Could you check a few things on this model? Use its own coordinates, in mm. A direction names the side the tool comes from. Give positions to 0.01 mm unless a question says otherwise; leave off trailing zeros. Write each loop counter-clockwise with the first axis right and the second up, starting at its lowest first coordinate (ties: lowest second). Pieces come first, ordered by that corner, then holes. Notation, with made-up numbers: (52.25, -30) - (91.25, -30) arc R19 ccw to (91.25, -4) - close; hole circle Ø6 at (-1.75, -32). An arc over 180 degrees is marked (long way). Write item = value, one per line.
from build123d import *

# Parameters (mm, degrees)
SKETCH_1_R          = 23
SKETCH_1_R_2        = 1.5
SKETCH_1_R_3        = 11.1
EXTRUDE_1_DEPTH     = 1.5
CUT_EXTRUDE_1_DEPTH = 33.56148031


with BuildPart() as part:
    # 草图1 → 凸台-拉伸1 (new body)
    with BuildSketch(Plane.XY):
        Circle(SKETCH_1_R)
        with Locations((0, 20)):
            Circle(SKETCH_1_R_2, mode=Mode.SUBTRACT)
        Circle(SKETCH_1_R_3, mode=Mode.SUBTRACT)
        with Locations((17.320508076, -10)):
            Circle(SKETCH_1_R_2, mode=Mode.SUBTRACT)
        with Locations((-17.320508076, -10)):
            Circle(SKETCH_1_R_2, mode=Mode.SUBTRACT)
    extrude(amount=EXTRUDE_1_DEPTH)

    # 草图2 → 切除-拉伸1 (cut, through all)
    with BuildSketch(Plane.XY.offset(1.5)):
        with BuildLine():
            ThreePointArc((-8.029746973, 17.219847954), (-16.454482672, 9.5), (-18.927699264, -1.655959112))
            ThreePointArc((-18.927699264, -1.655959112), (-16.815165904, -3.428585075), (-15.042539941, -1.316051715))
            ThreePointArc((-15.042539941, -1.316051715), (-13.076983597, 7.55), (-6.381535752, 13.685247584))
            ThreePointArc((-6.381535752, 13.685247584), (-5.438341178, 16.276653379), (-8.029746973, 17.219847954))
        make_face()
        with BuildLine():
            ThreePointArc((18.927699264, -1.655959112), (16.454482672, 9.5), (8.029746973, 17.219847954))
            ThreePointArc((8.029746973, 17.219847954), (5.438341178, 16.276653379), (6.381535752, 13.685247584))
            ThreePointArc((6.381535752, 13.685247584), (13.076983597, 7.55), (15.042539941, -1.316051715))
            ThreePointArc((15.042539941, -1.316051715), (16.815165904, -3.428585075), (18.927699264, -1.655959112))
        make_face()
        with BuildLine():
            ThreePointArc((-10.897952291, -15.563888841), (0, -19), (10.897952291, -15.563888841))
            ThreePointArc((10.897952291, -15.563888841), (11.376824726, -12.848068304), (8.661004189, -12.369195869))
            ThreePointArc((8.661004189, -12.369195869), (0, -15.1), (-8.661004189, -12.369195869))
            ThreePointArc((-8.661004189, -12.369195869), (-11.376824726, -12.848068304), (-10.897952291, -15.563888841))
        make_face()
    extrude(amount=-CUT_EXTRUDE_1_DEPTH, mode=Mode.SUBTRACT)


solid = part.part
1. For pin 1 (5 mm diameter, centred on x = 7, y = -1.5, fed in from +Z), with a flat end and sliding along its axis, tell me the tip position at first contact or that it passes through.
Filled sheet:
pin_1 = through
2. If we section it at A-A, the plane x = 0: Please give me the cut outline in (y, z), and give its area (4 significant figures).
Filled sheet:
outline = (-23, 0) - (-19, 0) - (-19, 1.5) - (-23, 1.5) - close; (-15.1, 0) - (-11.1, 0) - (-11.1, 1.5) - (-15.1, 1.5) - close; (11.1, 0) - (18.5, 0) - (18.5, 1.5) - (11.1, 1.5) - close; (21.5, 0) - (23, 0) - (23, 1.5) - (21.5, 1.5) - close
area = 25.35 mm2
3. If we section it at D-D, the plane z = 0.6: Please give me the cut outline in (x, y).
Filled sheet:
outline = circle Ø46 at (0, 0); hole (-18.93, -1.66) arc R1.95 ccw to (-15.04, -1.32) arc R15.1 cw to (-6.38, 13.69) arc R1.95 ccw to (-8.03, 17.22) arc R19 ccw to start; hole circle Ø3 at (-17.32, -10); hole circle Ø22.2 at (0, 0); hole (-10.9, -15.56) arc R19 ccw to (10.9, -15.56) arc R1.95 ccw to (8.66, -12.37) arc R15.1 cw to (-8.66, -12.37) arc R1.95 ccw to start; hole circle Ø3 at (0, 20); hole (6.38, 13.69) arc R15.1 cw to (15.04, -1.32) arc R1.95 ccw to (18.93, -1.66) arc R19 ccw to (8.03, 17.22) arc R1.95 ccw to start; hole circle Ø3 at (17.32, -10)
4. I need wall thicknesses on line 1 (Y direction, x = 0, z = 1.1); line 2 (Y direction, x = 9, z = 1.4); line 3 (Y direction, x = -2, z = 0.8). Which ranges of each line are inside material? Lowest first, please.
Filled sheet:
line_1 = -23 to -19, -15.1 to -11.1, 11.1 to 18.5, 21.5 to 23
line_2 = -21.17 to -16.73, -12.18 to -6.5, 6.5 to 12.12, 16.73 to 21.17
line_3 = -22.91 to -18.89, -14.97 to -10.92, 10.92 to 22.91
5. If we section it at B-B, the plane y = 0: Please give me the cut outline in (x, z), and give its area (3 significant figures).
Filled sheet:
outline = (-23, 0) - (-19, 0) - (-19, 1.5) - (-23, 1.5) - close; (-15.1, 0) - (-11.1, 0) - (-11.1, 1.5) - (-15.1, 1.5) - close; (11.1, 0) - (15.1, 0) - (15.1, 1.5) - (11.1, 1.5) - close; (19, 0) - (23, 0) - (23, 1.5) - (19, 1.5) - close
area = 24.0 mm2
6. If we section it at C-C, the plane y = -5: Please give me the cut outline in (x, z).
Filled sheet:
outline = (-22.45, 0) - (-9.91, 0) - (-9.91, 1.5) - (-22.45, 1.5) - close; (9.91, 0) - (22.45, 0) - (22.45, 1.5) - (9.91, 1.5) - close
7. Which directions (+Z, -Z, +X, -X, +Y, -Y) give clear straight access to the entire face, cutting with the end or side of a thin tool? Please do faces 1 (the face through (-5.4, -9.9, 1.5)), 2 (the face through (13.012, 7.662, 0.76)).
Filled sheet:
face_1 = +Z, +X, -X, +Y, -Y
face_2 = +Z, -Z
8. Thinking about a two-plate mould opening in X: for faces 3 (the face through (5.46, 16.32, 0.76)), 4 (the face through (-5.4, -9.9, 0)), 5 (the face through (-2.994, 22.804, 0.74)), which applies, pulls with the +X half, pulls with the -X half, needs draft (parallel to the pull), parting line crosses it, or undercut?
Filled sheet:
face_3 = undercut
face_4 = needs draft
face_5 = parting line crosses it
